Input: part model. Units: mm. Frame: model coordinates. A direction names the side the tool comes from. Give positions to 0.01 mm unless a question says otherwise; leave off trailing zeros. Loops run counter-clockwise (first coordinate to the right, second up) from the corner with the lowest first, then second, coordinate; pieces in that order, holes last. Notation, with made-up numbers: M -31,20.5 L -14,20.5 A16 ccw -14,25.5 Z; hole C 6,-13.5 d8. An arc over 180 degrees is marked long. Use CSV: the item, a comma, the result in double quotes. Start each with the question number.
Q1. Section C-C, the plane x = -34.5. Output: boundary loops of the cut face in (y, z), plus the area to 3 significant figures.
Q2. Reachability of faces 1 (the flat face through (1.45, -22, 1)), 2 (the flat face through (36, -27.71, 1)), 3 (the flat face through (-3.135, -25, 1)), 4 (the flat face through (8.043, 29, 2)) from +Z, -Z, +X, -X, +Y, -Y: full face, straight path, thin tool, end or side. Return the list, or none.
Q3. Section A-A, the plane x = 46.86. Output: boundary loops of the cut face in (y, z) (3 decimals).
Q4. Pin query (flat end, axial travel): pin 1 (2.5 mm diameter, centred on x = -46.86, y = 0.01, fed in from -Z); pin 2 (0.9 mm diameter, centred on y = -28.5, z = 1, fed in from -X); pin 3 (0.8 mm diameter, centred on x = -2.5, z = 2, fed in from +Y); pin 4 (1.3 mm diameter, centred on x = 2, z = 1.5, fed in from -Y). Return the tip coordinate at first contact, or that it passes through.
Q5. Material intervals for line 1 along Y through (x, z) = (-46.86, 1) (3 decimals); line 2 along Y through (x, z) = (-2, 1.75); line 3 along X through (y, z) = (24.5, 0.3) (3 decimals), sorted ascending.
Q6. Section B-B, the plane y = -12. Output: boundary loops of the cut face in (x, z), plus the area to 3 significant figures.
Q7. Pull-direction query (Y, two-part tool) for faces 5 (the flat face through (3.135, 25, 1)), 6 (the flat face through (24.13, 29, 2)), 7 (the flat face through (-16, 30.71, 1)); classes: released by +Y, released by -Y, zero draft, split by the parting line, or undercut.
from build123d import *

# Parameters (mm, degrees)
SKETCH1_W           = 96.52
SKETCH1_H           = 55.42
BOSS_EXTRUDE1_DEPTH = 3
SKETCH2_W           = 48.26
SKETCH2_H           = 3
BOSS_EXTRUDE2_DEPTH = 3
SKETCH4_W           = 3
SKETCH4_H           = 29.21
CUT_EXTRUDE1_DEPTH  = 3
SKETCH5_W           = 16.086666666
SKETCH5_H           = 3
CUT_EXTRUDE2_DEPTH  = 3
SKETCH6_W           = 3
SKETCH6_H           = 9.737913064
BOSS_EXTRUDE3_DEPTH = 3
SKETCH7_W           = 2.9
SKETCH7_H           = 3
CUT_EXTRUDE3_DEPTH  = 6.2
SKETCH9_W           = 6.27
SKETCH9_H           = 2.573555094
CUT_EXTRUDE4_DEPTH  = 3
SKETCH10_R          = 1.45
CUT_EXTRUDE5_DEPTH  = 3


with BuildPart() as part:
    # Sketch1 → Boss-Extrude1 (new body)
    with BuildSketch(Plane.XY):
        Rectangle(SKETCH1_W, SKETCH1_H)
    extrude(amount=BOSS_EXTRUDE1_DEPTH)

    # Sketch2 → Boss-Extrude2 (add)
    with BuildSketch(Plane(origin=(0, 27.71, 0), x_dir=(1, 0, 0), z_dir=(0, 1, 0))):
        with Locations((0, -1.5)):
            Rectangle(SKETCH2_W, SKETCH2_H)
    boss_extrude2 = extrude(amount=BOSS_EXTRUDE2_DEPTH)

    # Mirror1: Boss-Extrude2 across plane
    add(boss_extrude2.mirror(Plane.ZX))

    # Sketch4 → Cut-Extrude1 (cut)
    with BuildSketch(Plane(origin=(48.26, 0, 0), x_dir=(0, 0, -1), z_dir=(1, 0, 0))):
        with Locations((-1.5, 0)):
            Rectangle(SKETCH4_W, SKETCH4_H)
    cut_extrude1 = extrude(amount=-CUT_EXTRUDE1_DEPTH, mode=Mode.SUBTRACT)

    # Mirror2: Cut-Extrude1 across plane
    add(cut_extrude1.mirror(Plane(origin=(0, 0, 0), x_dir=(0, 0, 1), z_dir=(1, 0, 0))), mode=Mode.SUBTRACT)

    # Sketch5 → Cut-Extrude2 (cut)
    with BuildSketch(Plane(origin=(0, 30.71, 0), x_dir=(1, 0, 0), z_dir=(0, 1, 0))):
        with Locations((0, -1.5)):
            Rectangle(SKETCH5_W, SKETCH5_H)
    cut_extrude2 = extrude(amount=-CUT_EXTRUDE2_DEPTH, mode=Mode.SUBTRACT)

    # Mirror3: Cut-Extrude2 across plane
    add(cut_extrude2.mirror(Plane.ZX), mode=Mode.SUBTRACT)

    # Sketch6 → Boss-Extrude3 (add)
    with BuildSketch(Plane.ZY.offset(45.26)):
        with Locations((1.5, 0)):
            Rectangle(SKETCH6_W, SKETCH6_H)
    boss_extrude3 = extrude(amount=BOSS_EXTRUDE3_DEPTH)

    # Mirror4: Boss-Extrude3 across plane
    add(boss_extrude3.mirror(Plane(origin=(0, 0, 0), x_dir=(0, 0, 1), z_dir=(1, 0, 0))))

    # Sketch7 → Cut-Extrude3 (cut)
    with BuildSketch(Plane.XZ.offset(27.71)):
        with Locations((0, 1.5)):
            Rectangle(SKETCH7_W, SKETCH7_H)
    cut_extrude3 = extrude(amount=-CUT_EXTRUDE3_DEPTH, mode=Mode.SUBTRACT)

    # Sketch9 → Cut-Extrude4 (cut)
    with BuildSketch(Plane(origin=(0, 0, 0), x_dir=(-1, 0, 0), z_dir=(0, 0, -1))):
        with Locations((0, -24.61)):
            Rectangle(SKETCH9_W, SKETCH9_H)
    cut_extrude4 = extrude(amount=-CUT_EXTRUDE4_DEPTH, mode=Mode.SUBTRACT)

    # Mirror5: Cut-Extrude3 across plane
    add(cut_extrude3.mirror(Plane.ZX), mode=Mode.SUBTRACT)

    # Mirror6: Cut-Extrude4 across plane
    add(cut_extrude4.mirror(Plane.ZX), mode=Mode.SUBTRACT)

    # Sketch10 → Cut-Extrude5 (cut)
    with BuildSketch(Plane(origin=(0, 0, 0), x_dir=(-1, 0, 0), z_dir=(0, 0, -1))):
        with Locations((46.86, 0.006629449)):
            Circle(SKETCH10_R)
    cut_extrude5 = extrude(amount=-CUT_EXTRUDE5_DEPTH, mode=Mode.SUBTRACT)

    # Mirror7: Cut-Extrude5 across plane
    add(cut_extrude5.mirror(Plane(origin=(0, 0, 0), x_dir=(0, 0, 1), z_dir=(1, 0, 0))), mode=Mode.SUBTRACT)


solid = part.part
A:
1,outline,"M -27.71,0 L 27.71,0 L 27.71,3 L -27.71,3 Z"
1,area,"166 mm^2"
2,face 1,"+Z, -Z, -Y"
2,face 2,"+Z, -Z, +X, -Y"
2,face 3,"+Z, -Z"
2,face 4,"+Z, -Z, +Y"
3,outline,"M -27.71,0 L -14.605,0 L -14.605,3 L -27.71,3 Z; M -4.869,0 L -1.443,0 L -1.443,3 L -4.869,3 Z; M 1.457,0 L 4.869,0 L 4.869,3 L 1.457,3 Z; M 14.605,0 L 27.71,0 L 27.71,3 L 14.605,3 Z"
4,pin 1,"through"
4,pin 2,"x = -24.13"
4,pin 3,"y = 27.71"
4,pin 4,"y = -27.71"
5,line 1,"-27.71 to -14.605, -4.869 to -1.443, 1.457 to 4.869, 14.605 to 27.71"
5,line 2,"-27.71 to -25.9, -23.32 to 23.32, 25.9 to 27.71"
5,line 3,"-48.26 to -3.135, 3.135 to 48.26"
6,outline,"M -45.26,0 L 45.26,0 L 45.26,3 L -45.26,3 Z"
6,area,"272 mm^2"
7,face 5,"undercut"
7,face 6,"zero draft"
7,face 7,"released by +Y"
